Geometry check sheet. Reference: the model listing, model coordinates, mm. Face numbers are marked on the shaded views. A direction names the side the tool comes from. Give positions to 0.01 mm unless a question says otherwise; leave off trailing zeros. Order: outer loops, then holes, each group sorted by start corner. A loop starts at its lowest first (then second) coordinate and runs counter-clockwise, first axis right, second up. Notation, with made-up numbers: M -16.75,-6 L 29.25,-6 A14 ccw 29.25,13 Z; hole C 66,-14 d6. An arc over 180 degrees is marked long. Answer as a JSON object with one key per item and string values. Group by question number.
from build123d import *

# Parameters (mm, degrees)
CHAMFER1_SIZE = 1


with BuildPart() as part:
    # Sketch1 → Revolve1 (revolve)
    with BuildSketch(Plane(origin=(0, 0, 0), x_dir=(1, 0, 0), z_dir=(0, 1, 0))):
        Polygon((0, 0), (7, 0), (7, -3), (5, -3), (5, -28), (3, -28), (3, -44), (0, -44), align=None)
    revolve(axis=Axis((0, 0, 44), (0, 0, -1)))

    # Chamfer1
    chamfer1_edges = [part.edges().sort_by_distance(p)[0] for p in [
        (-3, 0, 44),
        (-5, 0, 28),
        (-7, 0, 3),
        (-7, 0, 0),
    ]]
    chamfer(chamfer1_edges, length=CHAMFER1_SIZE)


solid = part.part
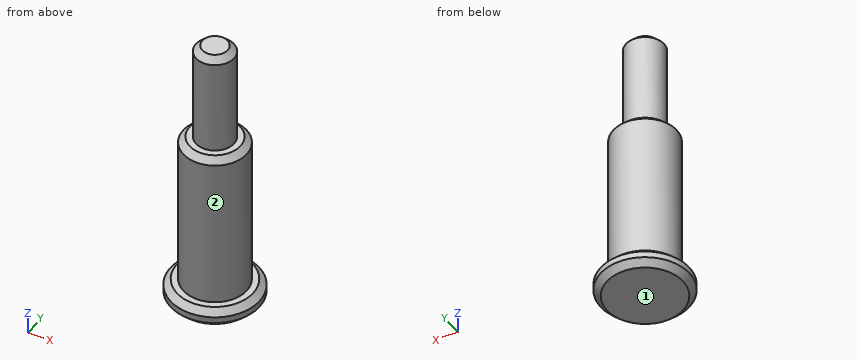
1. Thickness scan on line 1 along Z through (x, y) = (-3.5, 0); line 2 along Z through (x, y) = (1.5, 5.25); line 3 along X through (y, z) = (-2.5, 41.5). Record the ranges inside material, lowest first. Write a range as [from, to].
2. Cross-section at A-A (x = 0). Record the cut outline in (y, z).
3. Access from +Z, -Z, +X, -X, +Y, -Y to the whole of each face (thin tool, end or side, straight path). Record for the marked faces 1 and 2.
4. Cross-section at B-B (z = 38). Record the cut outline in (x, y).
5. Depth check by flat-ended pin: pin 1 (8 mm diameter, centred on y = 3.5, z = 31.5, fed in from -X); pin 2 (6 mm diameter, centred on y = -2.5, z = 19.5, fed in from -X); pin 3 (2 mm diameter, centred on x = -1.5, z = 18, fed in from -Y). Enter the tip coordinate at first touch or a pass-through.
6. Cross-section at C-C (z = 4). Record the cut outline in (x, y).
Report:
{
 "1": {"line 1": "z = [0, 28]", "line 2": "z = [0, 3]", "line 3": "x = [-1.66, 1.66]"},
 "2": {"outline": "M -7,1 L -6,0 L 6,0 L 7,1 L 7,2 L 6,3 L 5,3 L 5,27 L 4,28 L 3,28 L 3,43 L 2,44 L -2,44 L -3,43 L -3,28 L -4,28 L -5,27 L -5,3 L -6,3 L -7,2 Z"},
 "3": {"face 1": "-Z, +X, -X, +Y, -Y", "face 2": "+Z"},
 "4": {"outline": "C 0,0 d6"},
 "5": {"pin 1": "stops at x = -3.71", "pin 2": "stops at x = -5", "pin 3": "stops at y = -4.97"},
 "6": {"outline": "C 0,0 d10"}
}
